Geometry: final body of the model. Coordinates: model frame, mm. A direction names the side the tool comes from. Give positions to 0.01 mm unless a question says otherwise; leave off trailing zeros. Write each loop counter-clockwise with the first axis right and the second up, starting at its lowest first coordinate (ties: lowest second). Pieces come first, ordered by that corner, then holes. Notation, with made-up numbers: M 25,18 L 81,18 A26 cw 81,34 Z; hole C -35,18.25 d7. An arc over 180 degrees is marked long. One line per question, with ' | ' between items.
from build123d import *

# Parameters (mm, degrees)
SKETCH_1_W          = 66
SKETCH_1_H          = 30.5
SKETCH_1_W_2        = 58
SKETCH_1_H_2        = 22.5
EXTRUDE_1_DEPTH     = 27
SKETCH_2_W          = 66
SKETCH_2_H          = 30.5
EXTRUDE_2_DEPTH     = 3
SKETCH_3_R          = 4
CUT_EXTRUDE_1_DEPTH = 52.517321124
SKETCH_4_R          = 6
CUT_EXTRUDE_2_DEPTH = 11
SKETCH_5_W          = 4
SKETCH_5_H          = 30.5
CUT_EXTRUDE_3_DEPTH = 52.517321124
SKETCH_6_W          = 30.5
SKETCH_6_H          = 4.5
EXTRUDE_3_DEPTH     = 10
SKETCH_7_W          = 2
SKETCH_7_H          = 22.5
CUT_EXTRUDE_4_DEPTH = 10
SKETCH_8_W          = 30.5
SKETCH_8_H          = 4.5
EXTRUDE_4_DEPTH     = 10
SKETCH_9_W          = 2
SKETCH_9_H          = 22.5
CUT_EXTRUDE_5_DEPTH = 10
SKETCH_10_W         = 62
SKETCH_10_H         = 30.5
CUT_EXTRUDE_6_DEPTH = 4


with BuildPart() as part:
    # 草图1 → 凸台-拉伸1 (new body)
    with BuildSketch(Plane(origin=(0, 0, 0), x_dir=(1, 0, 0), z_dir=(0, 1, 0))):
        with Locations((4.387096774, -7.711693548)):
            Rectangle(SKETCH_1_W, SKETCH_1_H)
        with Locations((4.387096774, -7.711693548)):
            Rectangle(SKETCH_1_W_2, SKETCH_1_H_2, mode=Mode.SUBTRACT)
    extrude(amount=EXTRUDE_1_DEPTH)

    # 草图2 → 凸台-拉伸2 (add)
    with BuildSketch(Plane(origin=(0, 27, 0), x_dir=(1, 0, 0), z_dir=(0, 1, 0))):
        with Locations((4.387096774, -7.711693548)):
            Rectangle(SKETCH_2_W, SKETCH_2_H)
    extrude(amount=-EXTRUDE_2_DEPTH)

    # 草图3 → 切除-拉伸1 (cut, through all)
    with BuildSketch(Plane(origin=(0, 27, 0), x_dir=(1, 0, 0), z_dir=(0, 1, 0))):
        with Locations(Location((7.387096774, -7.711693548, 0), (0, 0, 270))):
            Circle(SKETCH_3_R)
    extrude(amount=-CUT_EXTRUDE_1_DEPTH, mode=Mode.SUBTRACT)

    # 草图4 → 切除-拉伸2 (cut)
    with BuildSketch(Plane.ZY.offset(-33.387096774)):
        with Locations((7.711693548, 16)):
            Circle(SKETCH_4_R)
    extrude(amount=-CUT_EXTRUDE_2_DEPTH, mode=Mode.SUBTRACT)

    # 草图5 → 切除-拉伸3 (cut, through all)
    with BuildSketch(Plane.XZ):
        with Locations((-26.612903226, 7.711693548)):
            Rectangle(SKETCH_5_W, SKETCH_5_H)
    extrude(amount=-CUT_EXTRUDE_3_DEPTH, mode=Mode.SUBTRACT)

    # 草图6 → 凸台-拉伸3 (add)
    with BuildSketch(Plane(origin=(37.387096774, 0, 0), x_dir=(0, 0, -1), z_dir=(1, 0, 0))):
        with Locations((-7.711693548, 24.75)):
            Rectangle(SKETCH_6_W, SKETCH_6_H)
    extrude(amount=EXTRUDE_3_DEPTH)

    # 草图7 → 切除-拉伸4 (cut)
    with BuildSketch(Plane.XZ.offset(-22.5)):
        with Locations((42.387096774, 7.711693548)):
            Rectangle(SKETCH_7_W, SKETCH_7_H)
    extrude(amount=-CUT_EXTRUDE_4_DEPTH, mode=Mode.SUBTRACT)

    # 草图8 → 凸台-拉伸4 (add)
    with BuildSketch(Plane.ZY.offset(24.612903226)):
        with Locations((7.711693548, 24.75)):
            Rectangle(SKETCH_8_W, SKETCH_8_H)
    extrude(amount=EXTRUDE_4_DEPTH)

    # 草图9 → 切除-拉伸5 (cut)
    with BuildSketch(Plane.XZ.offset(-22.5)):
        with Locations((-29.612903226, 7.711693548)):
            Rectangle(SKETCH_9_W, SKETCH_9_H)
    extrude(amount=-CUT_EXTRUDE_5_DEPTH, mode=Mode.SUBTRACT)

    # 草图10 → 切除-拉伸6 (cut)
    with BuildSketch(Plane.XZ):
        with Locations((6.387096774, 7.711693548)):
            Rectangle(SKETCH_10_W, SKETCH_10_H)
    extrude(amount=-CUT_EXTRUDE_6_DEPTH, mode=Mode.SUBTRACT)


solid = part.part
(1) Draft query along Z for faces 1 (the face through (35.359, 17.802, 13.435)), 2 (the face through (7, 15, -7.538)), 3 (the face through (-31, 22.5, 7)). Return one class per face: released by +Z, released by -Z, zero draft, split by the parting line, or undercut.
Working result:
face 1: undercut | face 2: released by -Z | face 3: zero draft
(2) Cut plane C-C, the plane x = -7. Return loops of the section in (y, z).
Working result:
outline: M 4,-7.54 L 27,-7.54 L 27,22.96 L 4,22.96 L 4,18.96 L 24,18.96 L 24,-3.54 L 4,-3.54 Z
(3) First-contact query: P1, Ø6, axis at x = 16.5, z = 3.5, coming from the -Y side; P2, Ø3, axis at y = 10, z = -5.5, coming from the -X side; P3, Ø1, axis at y = 11, z = 11.5, coming from the -X side. Flat tips, straight axial feed; report the tip coordinate or a pass-through.
Working result:
P1: stops at y = 24 | P2: stops at x = -24.61 | P3: stops at x = 33.39
(4) Cut plane A-A, the plane z = 17. Return loops of the section in (x, y), then the cut area to 3 significant figures.
Working result:
outline: M -34.61,22.5 L -30.61,22.5 L -30.61,27 L -34.61,27 Z; M -28.61,22.5 L -24.61,22.5 L -24.61,24 L 33.39,24 L 33.39,4 L 37.39,4 L 37.39,22.5 L 41.39,22.5 L 41.39,27 L -28.61,27 Z; M 43.39,22.5 L 47.39,22.5 L 47.39,27 L 43.39,27 Z | area: 338 mm^2
(5) Set-up query: faces 4 (the face through (-24.613, 13, -6)), 5 (the face through (41.387, 25, 8)), 6 (the face through (-24.613, 23, 8)). Return all of +Z, -Z, +X, -X, +Y, -Y with unobstructed straight access to the full face (end or side cutting, diameter ignored); none if empty.
Working result:
face 4: +Z, -Z, -X, -Y | face 5: +Y, -Y | face 6: -Y
(6) Cut plane D-D, the plane y = 7.25. Return loops of the section in (x, z).
Working result:
outline: M -24.61,-7.54 L 37.39,-7.54 L 37.39,22.96 L -24.61,22.96 L -24.61,18.96 L 33.39,18.96 L 33.39,-3.54 L -24.61,-3.54 Z
(7) Material intervals for L1, parallel to X at y = 24.5, z = 12.5; L2, parallel to Z at x = 33, y = 20.25; L3, parallel to Y at x = 2.5, z = 13, sorted ascending. Write a range as [from, to].
Working result:
L1: x = [-34.61, -30.61], [-28.61, 41.39], [43.39, 47.39] | L2: z = [-7.54, -3.54], [18.96, 22.96] | L3: y = [24, 27]
(8) Cut plane B-B, the plane y = 16. Return loops of the section in (x, z), then the cut area to 3 significant figures.
Working result:
outline: M -24.61,-7.54 L 37.39,-7.54 L 37.39,1.71 L 33.39,1.71 L 33.39,-3.54 L -24.61,-3.54 Z; M -24.61,18.96 L 33.39,18.96 L 33.39,13.71 L 37.39,13.71 L 37.39,22.96 L -24.61,22.96 Z | area: 538 mm^2
